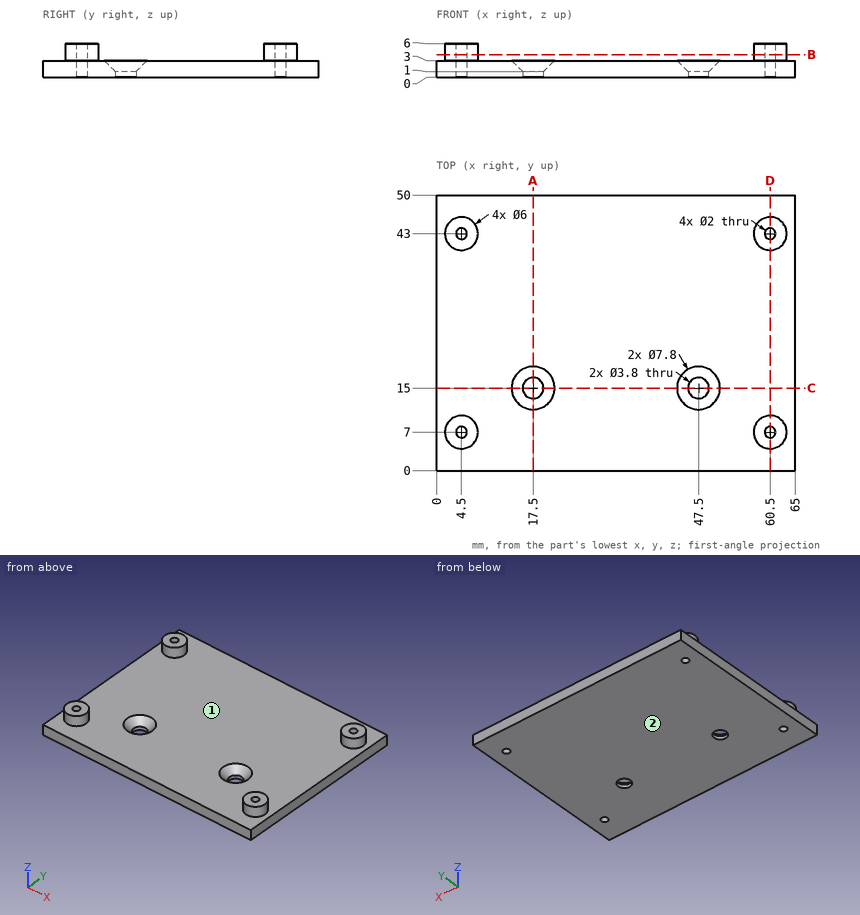
The drawing under review shows one solid part. Ordinate dimensions are in mm from its lowest x, y, z. Round coordinates to 2 decimals unless told otherwise and drop trailing zeros. Order: outer loops, then holes, each group sorted by start corner. A loop starts at its lowest first (then second) coordinate and runs counter-clockwise, first axis right, second up. Notation, with made-up numbers: (13.25, 44.25) -> (71.25, 44.25) arc R21 cw to (71.25, 64.25) -> close; hole circle Ø1 at (21, 68). An arc over 180 degrees is marked (long way). Return JSON: item names as keys, results as strings.
1. Take a section at B-B (z = 4.05). Write out the cut boundary in (x, y), then the cut area to 3 significant figures.
Answer block:
{"outline": "circle Ø6 at (4.5, 7); circle Ø6 at (4.5, 43); circle Ø6 at (60.5, 7); circle Ø6 at (60.5, 43); hole circle Ø2 at (4.5, 7); hole circle Ø2 at (4.5, 43); hole circle Ø2 at (60.5, 7); hole circle Ø2 at (60.5, 43)", "area": "101 mm²"}
2. The part is to be moulded in two halves that separate along X. For the marked faces 1 and 2, say which applies: +X half, -X half, draft (parallel to the pull), parting line (faces both ways), or undercut.
Answer block:
{"face 1": "undercut", "face 2": "draft"}
3. Take a section at D-D (x = 60.5). Write out the cut boundary in (y, z), then the cut area to 3 significant figures.
Answer block:
{"outline": "(0, 0) -> (6, 0) -> (6, 6) -> (4, 6) -> (4, 3) -> (0, 3) -> close; (8, 0) -> (42, 0) -> (42, 6) -> (40, 6) -> (40, 3) -> (10, 3) -> (10, 6) -> (8, 6) -> close; (44, 0) -> (50, 0) -> (50, 3) -> (46, 3) -> (46, 6) -> (44, 6) -> close", "area": "162 mm²"}
4. Insertion check: P1, Ø5, axis at x = 28, y = 33.5, coming from the +Z side. The pin has a flat end and moves straight along its axis. Give the tip position at first contact, or say it passes through.
Answer block:
{"P1": "stops at z = 3"}
5. Take a section at C-C (y = 15). Write out the cut boundary in (x, z).
Answer block:
{"outline": "(0, 0) -> (15.6, 0) -> (15.6, 1) -> (13.6, 3) -> (0, 3) -> close; (19.4, 0) -> (45.6, 0) -> (45.6, 1) -> (43.6, 3) -> (21.4, 3) -> (19.4, 1) -> close; (49.4, 0) -> (65, 0) -> (65, 3) -> (51.4, 3) -> (49.4, 1) -> close"}
6. For L1, parallel to Y at x = 4.5, z = 4.3; L2, parallel to Y at x = 4, z = 0.55; L3, parallel to X at y = 14, z = 2.3, list the stretches that pass through material, from the lowest coordinate up. Write a range as [from, to].
Answer block:
{"L1": "y = [4, 6], [8, 10], [40, 42], [44, 46]", "L2": "y = [0, 6.13], [7.87, 42.13], [43.87, 50]", "L3": "x = [0, 14.46], [20.54, 44.46], [50.54, 65]"}
7. Take a section at A-A (x = 17.5). Write out the cut boundary in (y, z), then the cut area to 3 significant figures.
Answer block:
{"outline": "(0, 0) -> (13.1, 0) -> (13.1, 1) -> (11.1, 3) -> (0, 3) -> close; (16.9, 0) -> (50, 0) -> (50, 3) -> (18.9, 3) -> (16.9, 1) -> close", "area": "135 mm²"}
